from build123d import *

# Parameters (mm, degrees)
SKETCH1_W             = 190
SKETCH1_H             = 25
SKETCH1_R             = 3.4
BASE_EXTRUDE_DEPTH    = 6
M8_TAPPED_HOLE1_D     = 6.8
M8_TAPPED_HOLE1_DEPTH = 22.25
M8_TAPPED_HOLE1_TIP   = 2.042926105


with BuildPart() as part:
    # Sketch1 → Base-Extrude (new body)
    with BuildSketch(Plane.XY):
        with Locations((-20, 0)):
            Rectangle(SKETCH1_W, SKETCH1_H)
        Circle(SKETCH1_R, mode=Mode.SUBTRACT)
        with Locations((-100, 0)):
            Circle(SKETCH1_R, mode=Mode.SUBTRACT)
    extrude(amount=BASE_EXTRUDE_DEPTH)

    # M8 Tapped Hole1
    with Locations(Plane(origin=(-100, 0, 6), x_dir=(1, 0, 0), z_dir=(0, 0, 1))):
        with Locations((0, 0), (100, 0)):
            Hole(M8_TAPPED_HOLE1_D / 2, depth=M8_TAPPED_HOLE1_DEPTH)
            with Locations((0, 0, -(M8_TAPPED_HOLE1_DEPTH + M8_TAPPED_HOLE1_TIP / 2))):  # 118° drill point
                Cone(0, M8_TAPPED_HOLE1_D / 2, M8_TAPPED_HOLE1_TIP, mode=Mode.SUBTRACT)


solid = part.part
Source: CAD feature listing. Evaluate the final solid. Frame: model axes, mm. Coordinates: 2 decimals unless noted, no trailing zeros. Order: outer loops, then holes, each group sorted by start corner. A loop starts at its lowest first (then second) coordinate and runs counter-clockwise, first axis right, second up.
Item 1: First-contact query: P1, Ø8, axis at x = -100, y = 0, coming from the -Z side. Flat tip, straight axial feed; report the tip coordinate or a pass-through.
Output values:
P1: stops at z = 0
Item 2: Material intervals for line 1 (X direction, y = 0.5, z = 1.45); line 2 (Y direction, x = -100, z = 3.35); line 3 (X direction, y = 1.5, z = 5.55), sorted ascending.
Output values:
line 1: x = -115 to -103.36, -96.64 to -3.36, 3.36 to 75
line 2: y = -12.5 to -3.4, 3.4 to 12.5
line 3: x = -115 to -103.05, -96.95 to -3.05, 3.05 to 75
Item 3: Cut plane B-B (y = 0). Return loops of the section in (x, z).
Output values:
outline: (-115, 0) - (-103.4, 0) - (-103.4, 6) - (-115, 6) - close; (-96.6, 0) - (-3.4, 0) - (-3.4, 6) - (-96.6, 6) - close; (3.4, 0) - (75, 0) - (75, 6) - (3.4, 6) - close
Item 4: Cut plane A-A (x = -100). Return loops of the section in (y, z).
Output values:
outline: (-12.5, 0) - (-3.4, 0) - (-3.4, 6) - (-12.5, 6) - close; (3.4, 0) - (12.5, 0) - (12.5, 6) - (3.4, 6) - close
Item 5: Cut plane C-C (z = 3.6). Return loops of the section in (x, y), plus the area to 3 significant figures.
Output values:
outline: (-115, -12.5) - (75, -12.5) - (75, 12.5) - (-115, 12.5) - close; hole circle Ø6.8 at (-100, 0); hole circle Ø6.8 at (0, 0)
area: 4,680 mm2
Item 6: Pull-direction query (Y, two-part tool) for faces 1 (the face through (75, 0, 3)), 2 (the face through (-0.74, -3.32, 2.96)), 3 (the face through (-21, 12.5, 3)), 4 (the face through (-103.4, 0.1, 3)); classes: pulls with the +Y half, pulls with the -Y half, needs draft (parallel to the pull), parting line crosses it, or undercut.
Output values:
face 1: needs draft
face 2: undercut
face 3: pulls with the +Y half
face 4: undercut
